```python
from build123d import *

# Parameters (mm, degrees)
SKETCH1_R                = 50
BOSS_EXTRUDE1_DEPTH      = 100
SKETCH2_W                = 25
SKETCH2_H                = 15
BOSS_EXTRUDE2_DEPTH      = 25
FILLET1_R                = 2.5
FILLET2_R                = 10
SKETCH3_R                = 5
CUT_EXTRUDE1_DEPTH       = 25
CIRPATTERN1_COUNT        = 2
FILLET1_OF_CIRPATTERN1_R = 2.5
FILLET2_OF_CIRPATTERN1_R = 10


with BuildPart() as part:
    # Sketch1 → Boss-Extrude1 (new body)
    with BuildSketch(Plane(origin=(0, 0, 0), x_dir=(1, 0, 0), z_dir=(0, 1, 0))):
        Circle(SKETCH1_R)
    extrude(amount=BOSS_EXTRUDE1_DEPTH)

    # Sketch2 → Boss-Extrude2 (add)
    with BuildSketch(Plane(origin=(0, 100, 0), x_dir=(1, 0, 0), z_dir=(0, 1, 0))):
        with Locations((0, -25)):
            Rectangle(SKETCH2_W, SKETCH2_H)
    boss_extrude2 = extrude(amount=BOSS_EXTRUDE2_DEPTH)

    # Fillet1
    fillet1_edges = [part.edges().sort_by_distance(p)[0] for p in [
        (12.5, 100, 25),
        (0, 100, 17.5),
        (-12.5, 100, 25),
        (0, 100, 32.5),
    ]]
    fillet(fillet1_edges, radius=FILLET1_R)

    # Fillet2
    fillet2_edges = [part.edges().sort_by_distance(p)[0] for p in [
        (12.5, 125, 25),
        (-12.5, 125, 25),
    ]]
    fillet(fillet2_edges, radius=FILLET2_R)

    # Sketch3 → Cut-Extrude1 (cut)
    with BuildSketch(Plane.XY.offset(32.5)):
        with Locations((0, 117.5)):
            Circle(SKETCH3_R)
    cut_extrude1 = extrude(amount=-CUT_EXTRUDE1_DEPTH, mode=Mode.SUBTRACT)

    # CirPattern1: Boss-Extrude2, Cut-Extrude1 ×2 about axis
    cirpattern1_axis = Axis((0, 0, 0), (0, 1, 0))
    for i in range(1, CIRPATTERN1_COUNT):
        add(boss_extrude2.rotate(cirpattern1_axis, i * 360 / CIRPATTERN1_COUNT))
        add(cut_extrude1.rotate(cirpattern1_axis, i * 360 / CIRPATTERN1_COUNT), mode=Mode.SUBTRACT)

    # Fillet1 of CirPattern1
    fillet1_of_cirpattern1_edges = [part.edges().sort_by_distance(p)[0] for p in [
        (-12.5, 100, -25),
        (0, 100, -17.5),
        (12.5, 100, -25),
        (0, 100, -32.5),
    ]]
    fillet(fillet1_of_cirpattern1_edges, radius=FILLET1_OF_CIRPATTERN1_R)

    # Fillet2 of CirPattern1
    fillet2_of_cirpattern1_edges = [part.edges().sort_by_distance(p)[0] for p in [
        (-12.5, 125, -25),
        (12.5, 125, -25),
    ]]
    fillet(fillet2_of_cirpattern1_edges, radius=FILLET2_OF_CIRPATTERN1_R)


solid = part.part
```
Model file for the job. Use its own axes, mm. A direction names the side the tool comes from. Coordinates: 2 decimals unless noted, no trailing zeros. Write each loop counter-clockwise with the first axis right and the second up, starting at its lowest first coordinate (ties: lowest second). Pieces come first, ordered by that corner, then holes. Notation, with made-up numbers: (-26, 54) - (-17, 54) arc R10 cw to (-17, 62) - close; hole circle Ø2 at (-7.75, 61.5). An arc over 180 degrees is marked (long way). One line per question, with ' | ' between items. Start each with the question number.
Q1. 3-axis set-ups, long thin cutter, end or side, ignore diameter. For faces 5 (the face through (0, 111, -32.5)), 6 (the face through (12.5, 109, 25)), 7 (the face through (0, 111, -17.5)), 8 (the face through (-12.5, 109, -25)): which of +Z, -Z, +X, -X, +Y, -Y reach the whole face in a straight line?
Q2. Cut at B-B, the plane y = 117.5. List the corners of the cut face in (x, z), then the cut area to 3 significant figures.
Q3. Cut at D-D, the plane z = 21. List the corners of the cut face in (x, y), then the cut area to 3 significant figures.
Q4. Cut at A-A, the plane x = 0. List the corners of the cut face in (y, z), then the cut area to 3 significant figures.
Q5. Pull direction Y, two halves, no side cores. Call faces 1 (the face through (0, 125, 25)), 2 (the face through (1.08, 112.62, -25.1)), 3 (the face through (-1.08, 112.62, 25.1)), 4 (the face through (-12.5, 109, 25)): pulls with the +Y half, pulls with the -Y half, needs draft (parallel to the pull), parting line crosses it, or undercut.
Q6. Cut at C-C, the plane z = 0. List the corners of the cut face in (x, y), then the cut area to 3 significant figures.
Q7. Drill centre lines: line 1 (Y direction, x = 0, z = 26.75); line 2 (Z direction, x = 1, y = 81.5); line 3 (Y direction, x = -22, z = -44). Where is each one in solid material? Low to high. Write a range as [from, to].
Q8. Pin check, flat tips, straight feed: pin 1 (12 mm diameter, centred on y = 69.5, z = 17, fed in from -X) (3 decimals); pin 2 (6 mm diameter, centred on x = 22, z = -13, fed in from +Y); pin 3 (14 mm diameter, centred on y = 110.5, z = -22.5, fed in from +X); pin 4 (6 mm diameter, centred on x = 0, y = 117.5, fed in from +Z). Stop position of each tip, or through.
Answer below:
1) face 5: -Z, +X, -X, +Y | face 6: +Z, -Z, +X, +Y | face 7: +X, -X, +Y | face 8: +Z, -Z, -X, +Y
2) outline: (-12.18, -32.5) - (-5, -32.5) - (-5, -17.5) - (-12.18, -17.5) - close; (-12.18, 17.5) - (-5, 17.5) - (-5, 32.5) - (-12.18, 32.5) - close; (5, -32.5) - (12.18, -32.5) - (12.18, -17.5) - (5, -17.5) - close; (5, 17.5) - (12.18, 17.5) - (12.18, 32.5) - (5, 32.5) - close | area: 431 mm^2
3) outline: (-45.38, 0) - (45.38, 0) - (45.38, 100) - (15, 100) arc R2.5 cw to (12.5, 102.5) - (12.5, 115) arc R10 ccw to (2.5, 125) - (-2.5, 125) arc R10 ccw to (-12.5, 115) - (-12.5, 102.5) arc R2.5 cw to (-15, 100) - (-45.38, 100) - close; hole circle Ø10 at (0, 117.5) | area: 9,580 mm^2
4) outline: (0, -50) - (100, -50) - (100, -35) arc R2.5 cw to (102.5, -32.5) - (112.5, -32.5) - (112.5, -17.5) - (102.5, -17.5) arc R2.5 cw to (100, -15) - (100, 15) arc R2.5 cw to (102.5, 17.5) - (112.5, 17.5) - (112.5, 32.5) - (102.5, 32.5) arc R2.5 cw to (100, 35) - (100, 50) - (0, 50) - close; (122.5, -32.5) - (125, -32.5) - (125, -17.5) - (122.5, -17.5) - close; (122.5, 17.5) - (125, 17.5) - (125, 32.5) - (122.5, 32.5) - close | area: 10,500 mm^2
5) face 1: pulls with the +Y half | face 2: undercut | face 3: undercut | face 4: needs draft
6) outline: (-50, 0) - (50, 0) - (50, 100) - (-50, 100) - close | area: 10,000 mm^2
7) line 1: [0, 112.5], [122.5, 125] | line 2: [-49.99, 49.99] | line 3: [0, 100]
8) pin 1: x = -48.775 | pin 2: y = 100 | pin 3: x = 12.5 | pin 4: through
